Source: CAD feature listing. Evaluate the final solid. Frame: model axes, mm. Give positions to 0.01 mm unless a question says otherwise; leave off trailing zeros. Order: outer loops, then holes, each group sorted by start corner. A loop starts at its lowest first (then second) coordinate and runs counter-clockwise, first axis right, second up. Notation, with made-up numbers: M -31.5,23 L -27.5,23 A28 cw -27.5,54 Z; hole C -26,59 d1. An arc over 180 degrees is marked long. Answer in a Markdown table with one row per item. Add a question column.
(1) Material intervals for line 1 along Y through (x, z) = (-29.5, 0.9); line 2 along Y through (x, z) = (31, 0.3), sorted ascending.
(2) Section query A-A, the plane z = 0.2. Return loops of the section in (x, y), plus the area to 3 significant figures.
(3) Section query C-C, the plane x = 11.5. Return loops of the section in (y, z).
(4) Section query B-B, the plane y = 16. Return loops of the section in (x, z), plus the area to 3 significant figures.
from build123d import *

# Parameters (mm, degrees)
F1_DEPTH = 1.058333


with BuildPart() as f1:
    # F0 (on Top) → F1 (new body)
    with BuildSketch(Plane.XY):
        Polygon((-40.879806, 12.7), (40.879447, 12.7), (-40.879806, 27.516667), align=None)
        Polygon((40.879806, -12.7), (40.879447, 12.7), (-40.879806, 12.7), (-40.879447, -12.7), align=None)
        Polygon((-40.879447, -27.516667), (40.879806, -12.7), (-40.879447, -12.7), align=None)
    extrude(amount=F1_DEPTH)


solid = f1.part
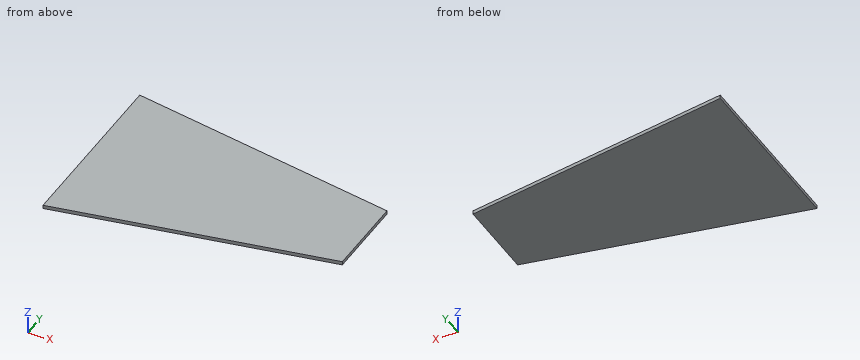
Values follow:
| question | item | result |
|---|---|---|
| 1 | line 1 | y = -25.45 to 25.45 |
| 1 | line 2 | y = -14.49 to 14.49 |
| 2 | outline | M -40.88,-27.52 L 40.88,-12.7 L 40.88,12.7 L -40.88,27.52 L -40.88,12.7 L -40.88,-12.7 Z |
| 2 | area | 3,290 mm² |
| 3 | outline | M -18.02,0 L 18.02,0 L 18.02,1.06 L -18.02,1.06 Z |
| 4 | outline | M -40.88,0 L 22.67,0 L 22.67,1.06 L -40.88,1.06 Z |
| 4 | area | 67.3 mm² |
